```python
from build123d import *

# Parameters (mm, degrees)
SKETCH1_R               = 4.826
BOSS_EXTRUDE1_DEPTH     = 3.3
SKETCH2_R               = 3.175
BOSS_EXTRUDE2_DEPTH     = 25.4
CUT_EXTRUDE1_DEPTH      = 10
CUT_EXTRUDE1_DEPTH_BACK = 10
SKETCH3_R               = 1.190625


with BuildPart() as part:
    # Sketch1 → Boss-Extrude1 (new body)
    with BuildSketch(Plane.XY):
        Circle(SKETCH1_R)
    extrude(amount=BOSS_EXTRUDE1_DEPTH)

    # Sketch2 → Boss-Extrude2 (add)
    with BuildSketch(Plane.XY.offset(3.3)):
        Circle(SKETCH2_R)
    extrude(amount=BOSS_EXTRUDE2_DEPTH)

    # Sketch3 → Cut-Extrude1 (cut, two sides: drawn at the far end of the back side and taken through both)
    with BuildSketch(Plane(origin=(0, 0, 0), x_dir=(1, 0, 0), z_dir=(0, 1, 0)).offset(-CUT_EXTRUDE1_DEPTH_BACK)):
        with Locations(Location((0, -25.13, 0), (0, 0, 90))):
            Circle(SKETCH3_R)
    extrude(amount=CUT_EXTRUDE1_DEPTH + CUT_EXTRUDE1_DEPTH_BACK, mode=Mode.SUBTRACT)


solid = part.part
```
Geometry check sheet. Reference: the model listing, model coordinates, mm. Give positions to 0.01 mm unless a question says otherwise; leave off trailing zeros. Order: outer loops, then holes, each group sorted by start corner. A loop starts at its lowest first (then second) coordinate and runs counter-clockwise, first axis right, second up.
1. Section check C-C, the plane z = 25.13. Enter the section's corners in (x, y) (3 decimals), and give its area (3 significant figures).
2. Section check A-A, the plane x = 0. Enter the section's corners in (y, z) (3 decimals).
3. Gauge pin test, flat ends, axial feed: pin 1 Ø5 at (y, z) = (2, 25) entering from -X (3 decimals); pin 2 Ø1 at (y, z) = (-1.5, 23.5) entering from -X; pin 3 Ø5 at (y, z) = (0.5, 3.5) entering from +X; pin 4 Ø1 at (y, z) = (2, 6.5) entering from +X. Record the tip position at first contact, or that the pin passes through.
4. Section check B-B, the plane y = 0. Enter the section's corners in (x, z) (3 decimals), and give its area (3 significant figures).
5. Thickness scan on L1, parallel to Z at x = -2.75, y = 2; L2, parallel to X at y = 0.75, z = 25.13; L3, parallel to Z at x = 0.25, y = -3. Record the ranges inside material, lowest first.
6. Release check for a two-part mould opening along Z. For faces 1 (the face through (0, 0, 0)), 2 (the face through (0, 0, 28.7)), 3 (the face through (0.724, -0.044, 26.075)), 4 (the face through (-3.83, -2.937, 1.627)) record: pulls with the +Z half, pulls with the -Z half, needs draft (parallel to the pull), parting line crosses it, or undercut.
7. Section check D-D, the plane x = -2.5. Enter the section's corners in (y, z).
Values follow:
1. outline: (-1.191, -2.943) - (-1.191, 2.943) arc R3.175 ccw to start; (1.191, -2.943) arc R3.175 ccw to (1.191, 2.943) - close
1. area: 16.9 mm2
2. outline: (-4.826, 0) - (4.826, 0) - (4.826, 3.3) - (3.175, 3.3) - (3.175, 23.939) - (-3.175, 23.939) - (-3.175, 3.3) - (-4.826, 3.3) - close; (-3.175, 26.321) - (3.175, 26.321) - (3.175, 28.7) - (-3.175, 28.7) - close
3. pin 1: stops at x = -3.175
3. pin 2: stops at x = -3.01
3. pin 3: stops at x = 4.83
3. pin 4: stops at x = 2.8
4. outline: (-4.826, 0) - (4.826, 0) - (4.826, 3.3) - (3.175, 3.3) - (3.175, 28.7) - (-3.175, 28.7) - (-3.175, 3.3) - (-4.826, 3.3) - close; hole circle Ø2.381 at (0, 25.13)
4. area: 189 mm2
5. L1: z = 0 to 3.3
5. L2: x = -3.09 to -1.19, 1.19 to 3.09
5. L3: z = 0 to 23.97, 26.29 to 28.7
6. face 1: pulls with the -Z half
6. face 2: pulls with the +Z half
6. face 3: undercut
6. face 4: needs draft
7. outline: (-4.13, 0) - (4.13, 0) - (4.13, 3.3) - (1.96, 3.3) - (1.96, 28.7) - (-1.96, 28.7) - (-1.96, 3.3) - (-4.13, 3.3) - close
